from build123d import *

# Parameters (mm, degrees)
BOSS_EXTRUDE1_DEPTH = 5.5
SKETCH3_OUTSIDE_W   = 39.986
SKETCH3_OUTSIDE_H   = 39.986
SKETCH3_OUTSIDE_R   = 6.5
CUT_EXTRUDE1_DEPTH  = 5.5
CUT_EXTRUDE1_DRAFT  = -45


with BuildPart() as part:
    # Sketch1 → Revolve1 (revolve)
    with BuildSketch(Plane.XY):
        with BuildLine():
            Line((0, 0), (-5, 0))
            Line((-5, 0), (-6, 1))
            Line((-6, 1), (-6, 10))
            ThreePointArc((-6, 10), (-5, 11), (-6, 12))
            Line((-6, 12), (-10, 12))
            Line((-10, 12), (-10, 15))
            Line((-10, 15), (0, 15))
            Line((0, 15), (0, 0))
        make_face()
    revolve(axis=Axis((0, 15, 0), (0, -1, 0)))

    # Sketch2 → Boss-Extrude1 (add)
    with BuildSketch(Plane(origin=(0, 15, 0), x_dir=(1, 0, 0), z_dir=(0, 1, 0))):
        Polygon((-3.75277675, 6.5), (-7.505553499, 0), (-3.75277675, -6.5), (3.75277675, -6.5), (7.505553499, 0), (3.75277675, 6.5), align=None)
    extrude(amount=BOSS_EXTRUDE1_DEPTH)


with BuildPart() as cut_extrude1_tool:
    # Sketch3 outside → Cut-Extrude1 (with draft: the straight prism first)
    with BuildSketch(Plane(origin=(0, 20.5, 0), x_dir=(1, 0, 0), z_dir=(0, 1, 0))):
        Rectangle(SKETCH3_OUTSIDE_W, SKETCH3_OUTSIDE_H)
        Circle(SKETCH3_OUTSIDE_R, mode=Mode.SUBTRACT)
    extrude(amount=-CUT_EXTRUDE1_DEPTH)
    # Cut-Extrude1: the draft: its side faces are tilted about the plane it starts from
    cut_extrude1_sides = [cut_extrude1_tool.faces().sort_by_distance(p)[0] for p in [
        (0, 17.75, 19.993),
        (19.993, 17.75, 0),
        (0, 17.75, -19.993),
        (-19.993, 17.75, 0),
        (-6.5, 17.75, 0),
    ]]
    draft(cut_extrude1_sides, Plane(origin=(0, 20.5, 0), x_dir=(1, 0, 0), z_dir=(0, 1, 0)), CUT_EXTRUDE1_DRAFT)


with BuildPart() as part_1:
    add(part.part)

    # Cut-Extrude1: cut by cut_extrude1_tool
    add(cut_extrude1_tool.part, mode=Mode.SUBTRACT)


solid = part_1.part
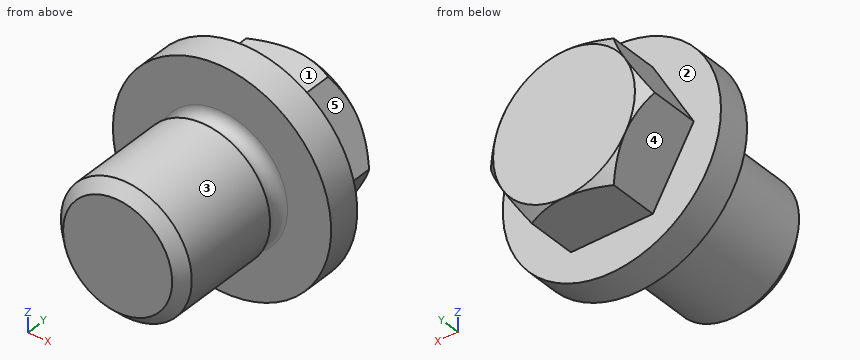
Check sheet for the modelled part. Datum: model origin and axes. Units: mm. Face numbers are marked on the shaded views. A direction names the side the tool comes from. Round coordinates to 2 decimals unless told otherwise and drop trailing zeros. Write each loop counter-clockwise with the first axis right and the second up, starting at its lowest first coordinate (ties: lowest second). Pieces come first, ordered by that corner, then holes. Notation, with made-up numbers: (-4, 24.5) -> (31, 24.5) arc R18 cw to (31, 44.5) -> close; hole circle Ø4 at (-8, -22.5). An arc over 180 degrees is marked (long way). Answer as CSV lines item,"result". Start each with the question number.
1) Tool access check on the marked faces 1, 2, 3, 4 and 5. Record the directions out of +Z, -Z, +X, -X, +Y, -Y that give a thin tool (end or side, any length) a straight path to the whole face; none if there is none.
2) Section check B-B on z = -8. Enter the section's corners in (x, y).
3) Section check A-A on y = 3.5. Enter the section's corners in (x, z).
4) Material ranges on line 1 (Y direction, x = -4.75, z = -8); line 2 (Y direction, x = -1.25, z = 5.25); line 3 (Y direction, x = -6, z = -2.5), recorded low to high. Write a range as from..to.
5) Go/stop test with flat-tipped pins: P1, Ø3, axis at y = 17, z = 6.5, coming from the -X side; P2, Ø1.5, axis at y = 12, z = -5, coming from the -X side; P3, Ø3, axis at x = -0.5, y = 19, coming from the +Z side. Record where each tip stops, or that it passes through.
Found:
1,face 1,"+Z, +X, -X, +Y"
1,face 2,"+Y"
1,face 3,"-Y"
1,face 4,"-Z, -X, +Y"
1,face 5,"+Z, +X, +Y"
2,outline,"(-6, 12) -> (6, 12) -> (6, 15) -> (-6, 15) -> close"
3,outline,"circle Ø12 at (0, 0)"
4,line 1,"y = 12..15"
4,line 2,"y = 0.4..10.2, 11.8..20.5"
4,line 3,"y = 12..20.5"
5,P1,"stops at x = -4.62"
5,P2,"stops at x = -9.05"
5,P3,"stops at z = 6.5"
